Geometry check sheet. Reference: drawing and pictorial views, mm from the part's lowest x, y, z. A direction names the side the tool comes from. Give positions to 0.01 mm unless a question says otherwise; leave off trailing zeros. Order: outer loops, then holes, each group sorted by start corner. A loop starts at its lowest first (then second) coordinate and runs counter-clockwise, first axis right, second up.
Item 1: Sectioned sample at B-B on y = 10.25. Record the boundary of the cut face in (x, z).
Item 2: Release check for a two-part mould opening along Y. For the marked faces 5, 6 and 7 record: released by +Y, released by -Y, zero draft, split by the parting line, or undercut.
Item 3: Sectioned sample at A-A on z = 1.6. Record the boundary of the cut face in (x, y).
Item 4: Access from +Z, -Z, +X, -X, +Y, -Y to the whole of each face (thin tool, end or side, straight path). Record for the marked faces 1, 2, 3 and 4.
Item 5: Gauge pin test, flat ends, axial feed: P1, Ø1, axis at y = 7.5, z = 3, coming from the +X side; P2, Ø2.5, axis at x = 5.5, z = 3, coming from the -Y side; P3, Ø0.7, axis at x = 5.5, z = 1.5, coming from the +Y side. Record the tip position at first contact, or that the pin passes through.
Item 6: Sectioned sample at D-D on z = 0.5. Record the boundary of the cut face in (x, y), and give its area (3 significant figures).
Item 7: Material ranges on line 1 along X through (y, z) = (9.5, 1.95); line 2 along Y through (x, z) = (4, 3.35), recorded low to high.
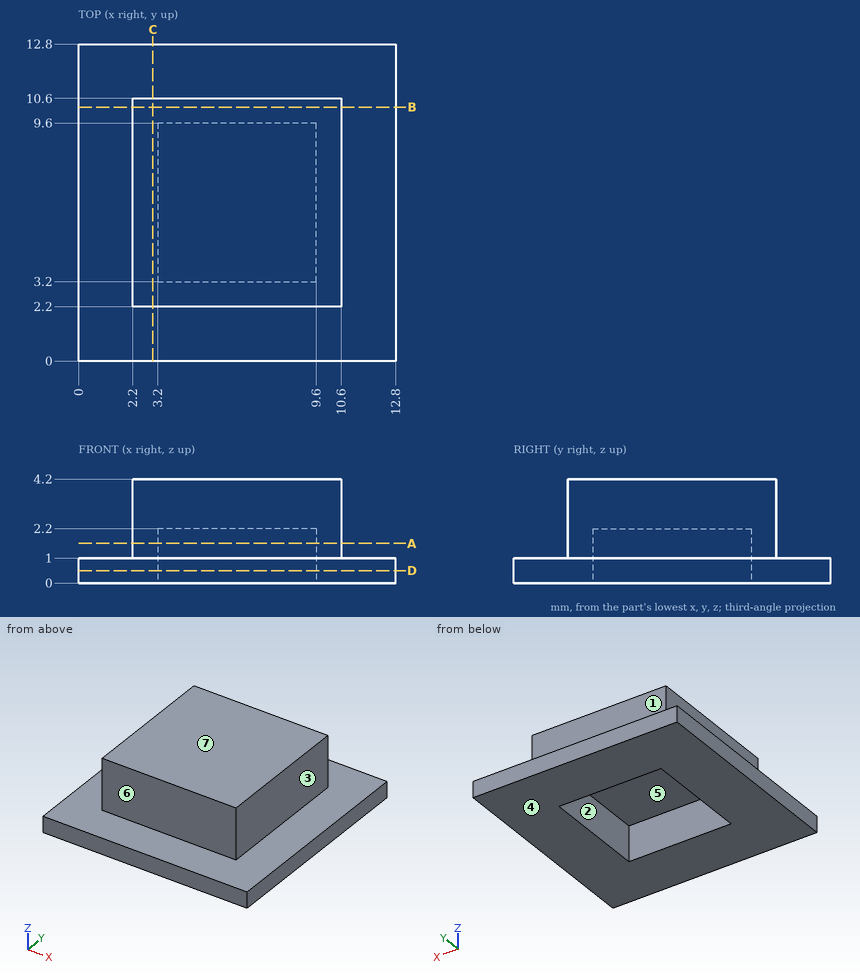
Report:
1. outline: (0, 0) - (12.8, 0) - (12.8, 1) - (10.6, 1) - (10.6, 4.2) - (2.2, 4.2) - (2.2, 1) - (0, 1) - close
2. face 5: undercut
2. face 6: released by -Y
2. face 7: zero draft
3. outline: (2.2, 2.2) - (10.6, 2.2) - (10.6, 10.6) - (2.2, 10.6) - close; hole (3.2, 3.2) - (9.6, 3.2) - (9.6, 9.6) - (3.2, 9.6) - close
4. face 1: +Z, +X, -X, +Y
4. face 2: -Z
4. face 3: +Z, +X, +Y, -Y
4. face 4: -Z, +X, -X, +Y, -Y
5. P1: stops at x = 10.6
5. P2: stops at y = 2.2
5. P3: stops at y = 10.6
6. outline: (0, 0) - (12.8, 0) - (12.8, 12.8) - (0, 12.8) - close; hole (3.2, 3.2) - (9.6, 3.2) - (9.6, 9.6) - (3.2, 9.6) - close
6. area: 123 mm2
7. line 1: x = 2.2 to 3.2, 9.6 to 10.6
7. line 2: y = 2.2 to 10.6
